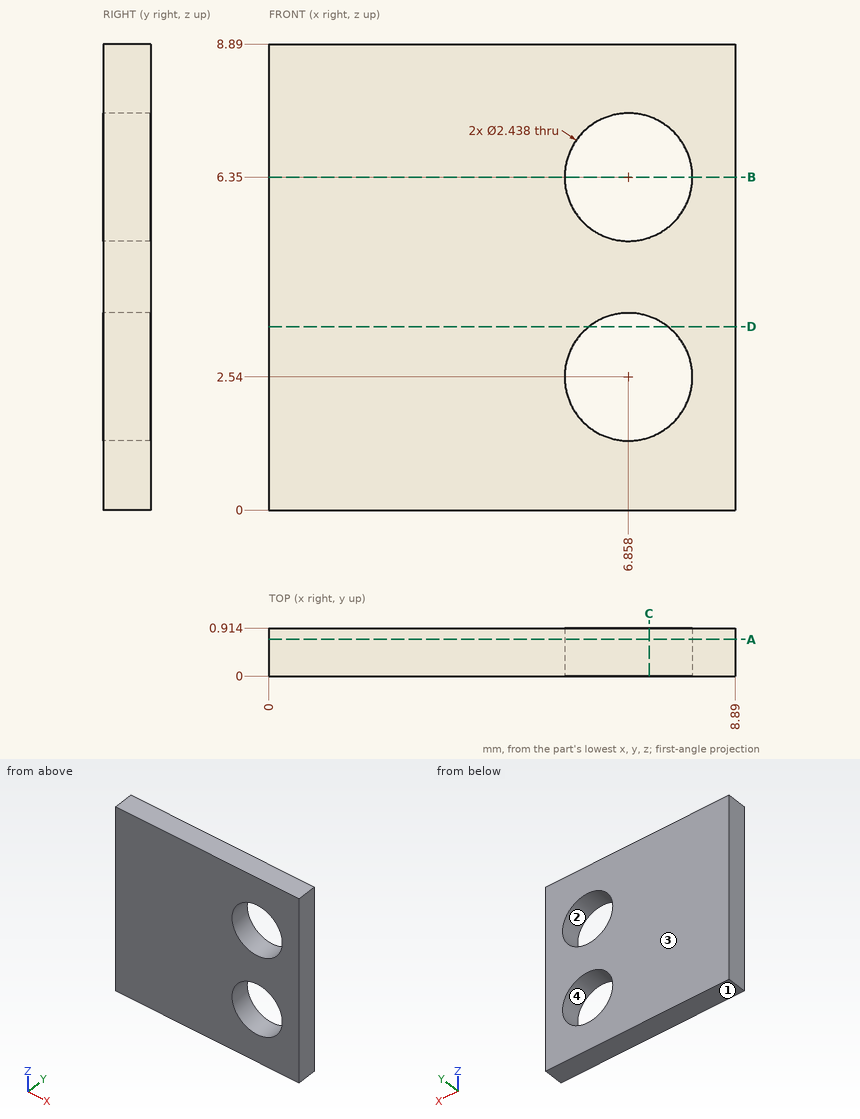
Verification items for this drawing (mm, ordinates from the low corner). Round coordinates to 2 decimals unless told otherwise and drop trailing zeros. Loops run counter-clockwise (first coordinate to the right, second up) from the corner with the lowest first, then second, coordinate; pieces in that order, holes last. Notation, with made-up numbers: (-37.5, 2) - (1.5, 2) arc R29 cw to (1.5, 23) - close; hole circle Ø7 at (76, -36.5). An arc over 180 degrees is marked (long way). Answer as CSV lines item,"result". Start each with the question number.
Item 1: Section check B-B (z = 6.35). Record the boundary of the cut face in (x, y) (1 decimal).
Item 2: Section check C-C (x = 7.25). Record the boundary of the cut face in (y, z) (1 decimal).
Item 3: Section check A-A (y = 0.7). Record the boundary of the cut face in (x, z), and give its area (3 significant figures).
Item 4: Scan lines: line 1 (X direction, y = 0.65, z = 3.5) (1 decimal); line 2 (Z direction, x = 6.25, y = 0.75); line 3 (X direction, y = 0.55, z = 6.5). Record each from-to range of solid material in increasing order. Write a range as [from, to].
Item 5: Release check for a two-part mould opening along Z. For the marked faces 1, 2, 3 and 4 record: +Z half, -Z half, draft (parallel to the pull), parting line (faces both ways), or undercut.
Item 6: Section check D-D (z = 3.5). Record the boundary of the cut face in (x, y) (1 decimal).
Report:
1,outline,"(0, 0) - (5.6, 0) - (5.6, 0.9) - (0, 0.9) - close; (8.1, 0) - (8.9, 0) - (8.9, 0.9) - (8.1, 0.9) - close"
2,outline,"(0, 0) - (0.9, 0) - (0.9, 1.4) - (0, 1.4) - close; (0, 3.7) - (0.9, 3.7) - (0.9, 5.2) - (0, 5.2) - close; (0, 7.5) - (0.9, 7.5) - (0.9, 8.9) - (0, 8.9) - close"
3,outline,"(0, 0) - (8.89, 0) - (8.89, 8.89) - (0, 8.89) - close; hole circle Ø2.44 at (6.86, 2.54); hole circle Ø2.44 at (6.86, 6.35)"
3,area,"69.7 mm2"
4,line 1,"x = [0, 6.1], [7.6, 8.9]"
4,line 2,"z = [0, 1.48], [3.6, 5.29], [7.41, 8.89]"
4,line 3,"x = [0, 5.65], [8.07, 8.89]"
5,face 1,"-Z half"
5,face 2,"undercut"
5,face 3,"draft"
5,face 4,"undercut"
6,outline,"(0, 0) - (6.1, 0) - (6.1, 0.9) - (0, 0.9) - close; (7.6, 0) - (8.9, 0) - (8.9, 0.9) - (7.6, 0.9) - close"
